Could you check a few things on this model? Use its own coordinates, in mm. A direction names the side the tool comes from. Round coordinates to 2 decimals unless told otherwise and drop trailing zeros. Loops run counter-clockwise (first coordinate to the right, second up) from the corner with the lowest first, then second, coordinate; pieces in that order, holes last. Notation, with made-up numbers: (-11.5, -26.75) - (-3.5, -26.75) arc R25 cw to (-3.5, 4.25) - close; hole circle Ø8 at (47, 63). An arc over 180 degrees is marked (long way). Answer as CSV lines item,"result". Start each with the question number.
1) Suppose I cut it at D-D, the plane z = -10.5. Write out the boundary of the cut face in (x, y).
2) We'd pull the mould along X, two halves only. Please class faces 1 (the face through (-29.5, 4, 0)), 2 (the face through (31.25, 4, 0)), 3 (the face through (0, -1.5, 0)): pulls with the +X half, pulls with the -X half, needs draft (parallel to the pull), parting line crosses it, or undercut.
3) I'm going to push flat-ended pins straight in: pin 1 Ø2 at (x, y) = (-8, 3) entering from -Z; pin 2 Ø1.4 at (x, y) = (-30, 5.5) entering from +Z; pin 3 Ø3.5 at (x, z) = (-8.5, -11.5) entering from +Y; pin 4 Ø11.5 at (x, z) = (2, -3) entering from +Y. Where does each tip first touch, or does it pass through?
4) Suppose I cut it at B-B, the plane y = 7.25. Write out the boundary of the cut face in (x, z).
5) Suppose I cut it at A-A, the plane z = 0. Write out the boundary of the cut face in (x, y).
6) Please list where these lines run through material, in increasing order: line 1 along X through (y, z) = (-1, 0); line 2 along X through (y, z) = (1.5, 9); line 3 along Z through (x, y) = (-18.7, -0.9).
7) Suppose I cut it at C-C, the plane x = 18.7. Write out the boundary of the cut face in (y, z), then the cut area to 4 significant figures.
8) Which directions (+Z, -Z, +X, -X, +Y, -Y) give clear straight access to the entire face, cutting with the end or side of a thin tool? Please do faces 4 (the face through (0, 1, -11.5)), 5 (the face through (30, 5, 9.95)), 6 (the face through (-30, 5, -9.95)), 7 (the face through (27.245, -0.74, 3.543)).
```python
from build123d import *

# Parameters (mm, degrees)
CROQUIS1_W              = 62.5
CROQUIS1_H              = 26.5
SALIENTE_EXTRUIR1_DEPTH = 1.5
CORTAR_EXTRUIR1_START   = 1.5
CROQUIS4_W              = 59
CROQUIS4_H              = 23
CORTAR_EXTRUIR1_DEPTH   = 1.5
CROQUIS5_R              = 9.25
CORTAR_EXTRUIR2_DEPTH   = 1.5
SALIENTE_EXTRUIR2_START = 31.25
CROQUIS6_W              = 19.9
CROQUIS6_H              = 10
SALIENTE_EXTRUIR2_DEPTH = 1.75
SALIENTE_EXTRUIR3_START = -31.25
CROQUIS6_3_W            = 19.9
CROQUIS6_3_H            = 10
SALIENTE_EXTRUIR3_DEPTH = 1.75


with BuildPart() as part:
    # Croquis1 → Saliente-Extruir1 (new body, symmetric)
    with BuildSketch(Plane(origin=(0, 0, 0), x_dir=(1, 0, 0), z_dir=(0, 1, 0))):
        Rectangle(CROQUIS1_W, CROQUIS1_H)
    extrude(amount=SALIENTE_EXTRUIR1_DEPTH, both=True)

    # Croquis4 → Cortar-Extruir1 (cut)
    with BuildSketch(Plane(origin=(0, 0, 0), x_dir=(1, 0, 0), z_dir=(0, 1, 0)).offset(CORTAR_EXTRUIR1_START)):
        Rectangle(CROQUIS4_W, CROQUIS4_H)
    extrude(amount=-CORTAR_EXTRUIR1_DEPTH, mode=Mode.SUBTRACT)

    # Croquis5 → Cortar-Extruir2 (cut)
    with BuildSketch(Plane(origin=(0, 0, 0), x_dir=(1, 0, 0), z_dir=(0, 1, 0))):
        with Locations((-18.7, 0)):
            Circle(CROQUIS5_R)
        with Locations((18.7, 0)):
            Circle(CROQUIS5_R)
    extrude(amount=-CORTAR_EXTRUIR2_DEPTH, mode=Mode.SUBTRACT)

    # Croquis6 → Saliente-Extruir2 (add)
    with BuildSketch(Plane(origin=(0, 0, 0), x_dir=(0, 0, -1), z_dir=(1, 0, 0)).offset(SALIENTE_EXTRUIR2_START)):
        with Locations((0, 3.5)):
            Rectangle(CROQUIS6_W, CROQUIS6_H)
    extrude(amount=-SALIENTE_EXTRUIR2_DEPTH)

    # Croquis6<3> → Saliente-Extruir3 (add)
    with BuildSketch(Plane(origin=(0, 0, 0), x_dir=(0, 0, -1), z_dir=(1, 0, 0)).offset(SALIENTE_EXTRUIR3_START)):
        with Locations((0, 3.5)):
            Rectangle(CROQUIS6_3_W, CROQUIS6_3_H)
    extrude(amount=SALIENTE_EXTRUIR3_DEPTH)


solid = part.part
```
Filled sheet:
1,outline,"(-31.25, -1.5) - (31.25, -1.5) - (31.25, 1.5) - (29.5, 1.5) - (29.5, 0) - (-29.5, 0) - (-29.5, 1.5) - (-31.25, 1.5) - close"
2,face 1,"undercut"
2,face 2,"pulls with the +X half"
2,face 3,"needs draft"
3,pin 1,"through"
3,pin 2,"z = 9.95"
3,pin 3,"y = 1.5"
3,pin 4,"y = 0"
4,outline,"(-31.25, -9.95) - (-29.5, -9.95) - (-29.5, 9.95) - (-31.25, 9.95) - close; (29.5, -9.95) - (31.25, -9.95) - (31.25, 9.95) - (29.5, 9.95) - close"
5,outline,"(-31.25, -1.5) - (-27.95, -1.5) - (-27.95, 0) - (-29.5, 0) - (-29.5, 8.5) - (-31.25, 8.5) - close; (-9.45, -1.5) - (9.45, -1.5) - (9.45, 0) - (-9.45, 0) - close; (27.95, -1.5) - (31.25, -1.5) - (31.25, 8.5) - (29.5, 8.5) - (29.5, 0) - (27.95, 0) - close"
6,line 1,"-31.25 to -27.95, -9.45 to 9.45, 27.95 to 31.25"
6,line 2,"-31.25 to -29.5, 29.5 to 31.25"
6,line 3,"-13.25 to -9.25, 9.25 to 13.25"
7,outline,"(-1.5, -13.25) - (1.5, -13.25) - (1.5, -11.5) - (0, -11.5) - (0, -9.25) - (-1.5, -9.25) - close; (-1.5, 9.25) - (0, 9.25) - (0, 11.5) - (1.5, 11.5) - (1.5, 13.25) - (-1.5, 13.25) - close"
7,area,"17.25 mm²"
8,face 4,"+Y"
8,face 5,"+Z, +X, -X, +Y"
8,face 6,"-Z, +X, -X, +Y"
8,face 7,"+Y, -Y"
